Can you work these out from the model? Positions are in its coordinate system, mm. A direction names the side the tool comes from. Coordinates: 2 decimals unless noted, no trailing zeros. Loops run counter-clockwise (first coordinate to the right, second up) from the corner with the lowest first, then second, coordinate; pieces in that order, holes last.
```python
from build123d import *

# Parameters (mm, degrees)
F1_DEPTH = 25.4
F2_R     = 6.35
F3_DEPTH = 12.701
F5_DEPTH = 25.401
F6_R     = 5.08
F7_R     = 5.08


with BuildPart() as f1:
    # F0 (on Front) → F1 (new body)
    with BuildSketch(Plane.XZ):
        Polygon((-40.276536, 60.90298), (-65.676536, 60.90298), (-65.676536, 10.10298), (9.114186, 10.10298), (9.114186, 22.80298), (-40.276536, 22.80298), align=None)
    extrude(amount=F1_DEPTH)

    # F2 (on face) → F3 (cut, through all)
    with BuildSketch(Plane.XY.offset(22.80298)):
        with Locations((-27.576536, -12.7)):
            Circle(F2_R)
        with Locations((-3.585814, -12.7)):
            Circle(F2_R)
        with BuildLine():
            ThreePointArc((0, 0), (8.89883, -12.7), (0, -25.4))
            Line((0, -25.4), (9.114186, -25.4))
            Line((9.114186, -25.4), (9.114186, 0))
            Line((9.114186, 0), (0, 0))
        make_face()
    extrude(amount=-F3_DEPTH, mode=Mode.SUBTRACT)

    # F4 (on face) → F5 (cut, through all)
    with BuildSketch(Plane.YZ.offset(-40.276536)):
        with BuildLine():
            ThreePointArc((-19.05, 48.20298), (-12.7, 41.85298), (-6.35, 48.20298))
            ThreePointArc((-6.35, 48.20298), (-12.7, 54.55298), (-19.05, 48.20298))
        make_face()
        with BuildLine():
            ThreePointArc((-19.05, 48.20298), (-12.7, 54.55298), (-6.35, 48.20298))
            Line((-6.35, 48.20298), (-6.35, 60.90298))
            Line((-6.35, 60.90298), (-19.05, 60.90298))
            Line((-19.05, 60.90298), (-19.05, 48.20298))
        make_face()
    extrude(amount=-F5_DEPTH, mode=Mode.SUBTRACT)

    # F6
    f6_edges = [f1.edges().sort_by_distance(p)[0] for p in [
        (-52.976536, -25.4, 60.90298),
    ]]
    fillet(f6_edges, radius=F6_R)

    # F7
    f7_edges = [f1.edges().sort_by_distance(p)[0] for p in [
        (-52.976536, 0, 60.90298),
    ]]
    fillet(f7_edges, radius=F7_R)


solid = f1.part
```
(1) If we mould it in two halves opening along X, with no side actions, what happens to faces 1 (the cylindrical face through (-4.96, -18.9, 16.54)), 2 (the cylindrical face through (-53.154, -1.449, 59.375)), 3 (the cylindrical face through (8.897, -12.469, 16.542))? For each: released by +X, released by -X, zero draft, split by the parting line, or undercut.
Check values:
face 1: undercut
face 2: zero draft
face 3: released by +X
(2) I want a section at D-D on y = -4.25. Write out the boundary of the cut face in (x, z), then the cut area to 3 significant figures.
Check values:
outline: (-65.68, 10.1) - (5.93, 10.1) - (5.93, 22.8) - (-40.28, 22.8) - (-40.28, 60.83) - (-65.68, 60.83) - close
area: 1,880 mm2
(3) I want a section at A-A on y = -12.7. Write out the boundary of the cut face in (x, z), then the cut area to 3 significant figures.
Check values:
outline: (-65.68, 10.1) - (-33.93, 10.1) - (-33.93, 22.8) - (-40.28, 22.8) - (-40.28, 41.85) - (-65.68, 41.85) - close; (-21.23, 10.1) - (-9.94, 10.1) - (-9.94, 22.8) - (-21.23, 22.8) - close; (2.76, 10.1) - (8.9, 10.1) - (8.9, 22.8) - (2.76, 22.8) - close
area: 1,110 mm2
(4) If I drill on probe 1 along Z at (x, y) = (-34.5, -7.75); probe 2 along Y at (x, z) = (-46.5, 50); probe 3 along X at (y, z) = (-7.75, 13), over which ranges is the centre line in solid material (lowest first)?
Check values:
probe 1: z = 10.1 to 22.8
probe 2: y = -25.4 to -19.05, -6.35 to 0
probe 3: x = -65.68 to -31.55, -23.6 to -7.56, 0.39 to 7.96
(5) I want a section at C-C on x = -43.5. Write out the boundary of the cut face in (y, z).
Check values:
outline: (-25.4, 10.1) - (0, 10.1) - (0, 55.82) arc R5.08 ccw to (-5.08, 60.9) - (-6.35, 60.9) - (-6.35, 48.2) arc R6.35 cw to (-19.05, 48.2) - (-19.05, 60.9) - (-20.32, 60.9) arc R5.08 ccw to (-25.4, 55.82) - close
(6) I want a section at B-B on x = -5. Write out the boundary of the cut face in (y, z).
Check values:
outline: (-25.4, 10.1) - (-18.89, 10.1) - (-18.89, 22.8) - (-25.4, 22.8) - close; (-6.51, 10.1) - (0, 10.1) - (0, 22.8) - (-6.51, 22.8) - close
(7) Which directions (+Z, -Z, +X, -X, +Y, -Y) give clear straight access to the entire face, cutting with the end or side of a thin tool? Please do faces 4 (the flat face through (-15, -13, 22.803)), 5 (the flat face through (-37, -13, 10.103)), 6 (the flat face through (-53, -19.05, 55)).
Check values:
face 4: +Z, +X, +Y, -Y
face 5: -Z, +X, -X, +Y, -Y
face 6: +Z, +X, -X
(8) I'm going to push flat-ended pins straight in: pin 1 (14.5 mm diameter, centred on x = -27.58, y = -12.7, fed in from -Z); pin 2 (1 mm diameter, centred on y = -5, z = 47.5, fed in from +X); pin 3 (3 mm diameter, centred on x = -13.5, y = -17, fed in from +Z). Where does each tip first touch, or does it pass through?
Check values:
pin 1: stops at z = 10.1
pin 2: stops at x = -40.28
pin 3: stops at z = 22.8
